Could you check a few things on this drawing? It's one solid part, dimensions in mm from its lowest x, y, z. A direction names the side the tool comes from. Round coordinates to 2 decimals unless told otherwise and drop trailing zeros. Write each loop counter-clockwise with the first axis right and the second up, starting at its lowest first coordinate (ties: lowest second). Pieces come first, ordered by that corner, then holes. Notation, with made-up numbers: (-16, 16.25) -> (43, 16.25) arc R27 cw to (43, 41.25) -> close; hole circle Ø11 at (-4, -21.5). An arc over 180 degrees is marked (long way). Answer in a Markdown table with one row per item. Add a question column.
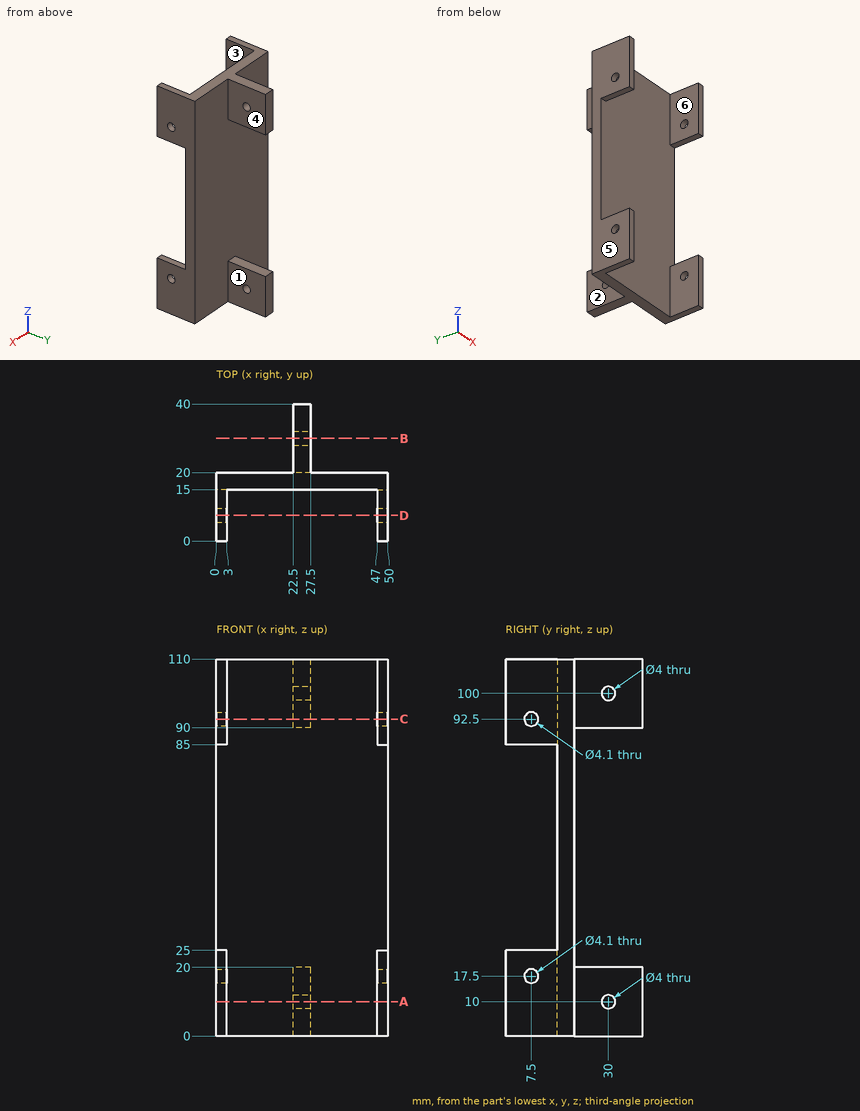
(1) I need wall thicknesses on L1, parallel to Z at x = 2, y = 10; L2, parallel to Z at x = 24, y = 24; L3, parallel to Y at x = 37, z = 73.5. Which ranges of each line are inside material? Lowest first, please.
(2) Suppose I cut it at C-C, the plane z = 92.5. Please give me the cut outline in (x, y), then the cut area to 3 significant figures.
(3) On a 3-axis mill with a long thin cutter (end or side, diameter ignored), from which of +Z, -Z, +X, -X, +Y, -Y can I reach the whole of each face in a straight line? I mean the marked faces 4, 5 and 6. Say none if no direction works.
(4) If we mould it in two halves opening along X, with no side actions, what happens to the marked faces 1, 2 and 3? For each: pulls with the +X half, pulls with the -X half, needs draft (parallel to the pull), parting line crosses it, or undercut.
(5) Suppose I cut it at D-D, the plane y = 7.5. State how many separate pieces and enclosed holes the cut face has, then the cut area to 3 significant figures.
(6) For P1, Ø4, axis at x = 43, z = 35, coming from the +Y side; P2, Ø10, axis at y = 34, z = 102.5, coming from the +X side; P3, Ø5, axis at y = 30, z = 100, coming from the -X side, each with a flat end and sliding along its axis, tell me the tip position at first contact or that it passes through.
(7) Suppose I cut it at B-B, the plane y = 30. Please give me the cut outline in (x, z), then the cut area to 3 significant figures.
(8) Suppose I cut it at A-A, the plane z = 10. Please give me the cut outline in (x, y), then the cut area to 3 significant figures.
Response:
| question | item | result |
|---|---|---|
| 1 | L1 | 0 to 25, 85 to 110 |
| 1 | L2 | 0 to 20, 90 to 110 |
| 1 | L3 | 15 to 20 |
| 2 | outline | (0, 0) -> (3, 0) -> (3, 5.45) -> (0, 5.45) -> close; (0, 9.55) -> (3, 9.55) -> (3, 15) -> (47, 15) -> (47, 9.55) -> (50, 9.55) -> (50, 20) -> (27.5, 20) -> (27.5, 40) -> (22.5, 40) -> (22.5, 20) -> (0, 20) -> close; (47, 0) -> (50, 0) -> (50, 5.45) -> (47, 5.45) -> close |
| 2 | area | 415 mm² |
| 3 | face 4 | +Z, -Z, +X, +Y |
| 3 | face 5 | +Z, -Z, -X, +Y, -Y |
| 3 | face 6 | +Z, -Z, -Y |
| 4 | face 1 | pulls with the +X half |
| 4 | face 2 | pulls with the -X half |
| 4 | face 3 | undercut |
| 5 | separate pieces | 8 |
| 5 | enclosed holes | 0 |
| 5 | area | 251 mm² |
| 6 | P1 | y = 20 |
| 6 | P2 | x = 27.5 |
| 6 | P3 | x = 22.5 |
| 7 | outline | (22.5, 0) -> (27.5, 0) -> (27.5, 8) -> (22.5, 8) -> close; (22.5, 12) -> (27.5, 12) -> (27.5, 20) -> (22.5, 20) -> close; (22.5, 90) -> (27.5, 90) -> (27.5, 98) -> (22.5, 98) -> close; (22.5, 102) -> (27.5, 102) -> (27.5, 110) -> (22.5, 110) -> close |
| 7 | area | 160 mm² |
| 8 | outline | (0, 0) -> (3, 0) -> (3, 15) -> (47, 15) -> (47, 0) -> (50, 0) -> (50, 20) -> (27.5, 20) -> (27.5, 28) -> (22.5, 28) -> (22.5, 20) -> (0, 20) -> close; (22.5, 32) -> (27.5, 32) -> (27.5, 40) -> (22.5, 40) -> close |
| 8 | area | 420 mm² |
